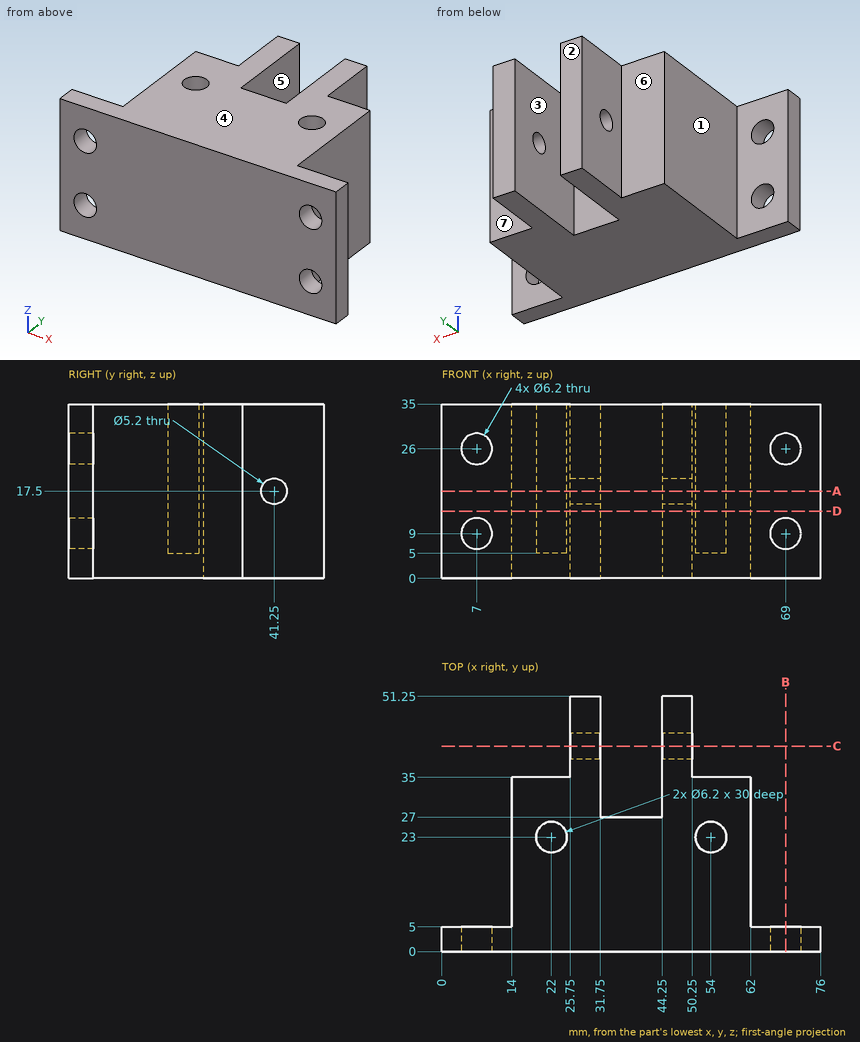
Can you work these out from the drawing? Everything is in mm from the part's minimum corner. A direction names the side the tool comes from. Coordinates: 2 decimals unless noted, no trailing zeros. Loops run counter-clockwise (first coordinate to the right, second up) from the corner with the lowest first, then second, coordinate; pieces in that order, holes last.
1. Imagine slicing it at B-B, the plane x = 69. Please give me the cut outline in (y, z).
2. For the marked faces 4, 5, 6 and 7, which set-ups out of +Z, -Z, +X, -X, +Y, -Y let a thin tool reach every point of the face, with its end or its side?
3. If we mould it in two halves opening along X, with no side actions, what happens to the marked faces 1, 2 and 3? For each: pulls with the +X half, pulls with the -X half, needs draft (parallel to the pull), parting line crosses it, or undercut.
4. I need wall thicknesses on L1, parallel to Z at x = 7, y = 1.75; L2, parallel to X at y = 23, z = 12.75; L3, parallel to X at y = 41, z = 12.5. Which ranges of each line are inside material? Lowest first, please.
5. Imagine slicing it at D-D, the plane z = 13.5. Please give me the cut outline in (x, y).
6. Imagine slicing it at A-A, the plane z = 17.5. Please give me the cut outline in (x, y), and give its area (3 significant figures).
7. Imagine slicing it at C-C, the plane y = 41.25. Please give me the cut outline in (x, z).
8. For P1, Ø8.5, axis at y = 41.25, z = 17.5, coming from the +X side; P2, Ø15, axis at y = 13.5, z = 18, coming from the -X side; P3, Ø7, axis at x = 69, z = 26, coming from the +Y side, each with a flat end and sliding along its axis, tell me the tip position at first contact or that it passes through.
Taken from the geometry:
1. outline: (0, 0) - (5, 0) - (5, 5.9) - (0, 5.9) - close; (0, 12.1) - (5, 12.1) - (5, 22.9) - (0, 22.9) - close; (0, 29.1) - (5, 29.1) - (5, 35) - (0, 35) - close
2. face 4: +Z, +X, -X, +Y, -Y
2. face 5: +Z, -Z, +Y
2. face 6: +Z, -Z, -X, +Y
2. face 7: +Z, -Z, +X, +Y
3. face 1: pulls with the -X half
3. face 2: needs draft
3. face 3: undercut
4. L1: z = 0 to 5.9, 12.1 to 22.9, 29.1 to 35
4. L2: x = 14 to 18.9, 25.1 to 50.9, 57.1 to 62
4. L3: x = 25.75 to 31.75, 44.25 to 50.25
5. outline: (0, 0) - (76, 0) - (76, 5) - (62, 5) - (62, 35) - (50.25, 35) - (50.25, 51.25) - (44.25, 51.25) - (44.25, 27) - (31.75, 27) - (31.75, 51.25) - (25.75, 51.25) - (25.75, 35) - (14, 35) - (14, 5) - (0, 5) - close; hole circle Ø6.2 at (22, 23); hole circle Ø6.2 at (54, 23)
6. outline: (0, 0) - (76, 0) - (76, 5) - (62, 5) - (62, 35) - (50.25, 35) - (50.25, 38.65) - (44.25, 38.65) - (44.25, 27) - (31.75, 27) - (31.75, 38.65) - (25.75, 38.65) - (25.75, 35) - (14, 35) - (14, 5) - (0, 5) - close; (25.75, 43.85) - (31.75, 43.85) - (31.75, 51.25) - (25.75, 51.25) - close; (44.25, 43.85) - (50.25, 43.85) - (50.25, 51.25) - (44.25, 51.25) - close; hole circle Ø6.2 at (22, 23); hole circle Ø6.2 at (54, 23)
6. area: 1,790 mm2
7. outline: (25.75, 0) - (31.75, 0) - (31.75, 14.9) - (25.75, 14.9) - close; (25.75, 20.1) - (31.75, 20.1) - (31.75, 35) - (25.75, 35) - close; (44.25, 0) - (50.25, 0) - (50.25, 14.9) - (44.25, 14.9) - close; (44.25, 20.1) - (50.25, 20.1) - (50.25, 35) - (44.25, 35) - close
8. P1: stops at x = 50.25
8. P2: stops at x = 14
8. P3: stops at y = 5
